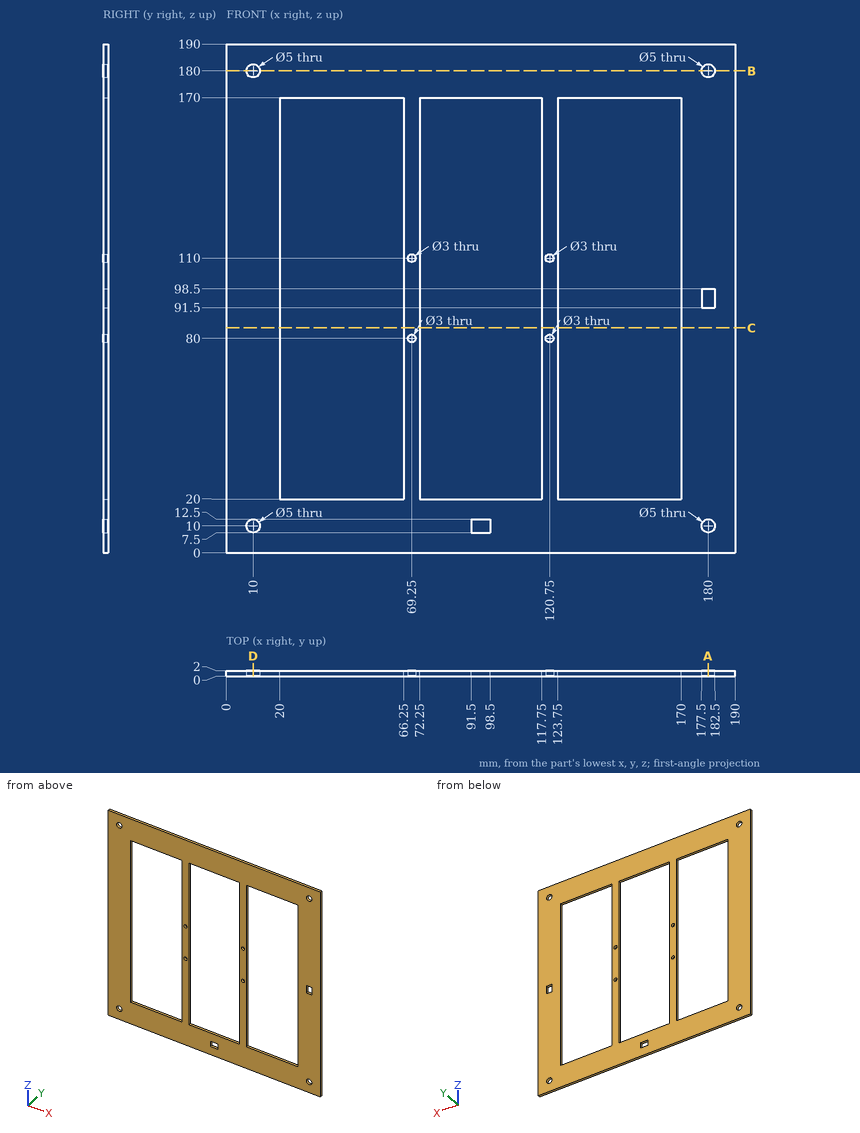
The figure shows three views and two pictorial views of one solid part (mm, origin at its lowest corner). Answer the questions. Give positions to 0.01 mm unless a question says otherwise; leave off trailing zeros. Loops run counter-clockwise (first coordinate to the right, second up) from the corner with the lowest first, then second, coordinate; pieces in that order, holes last. Notation, with made-up numbers: (43.25, -25) -> (75.25, -25) arc R23 cw to (75.25, -2) -> close; hole circle Ø8 at (62, -6.5). An arc over 180 degrees is marked (long way). Use a Markdown table: item, result. Add a question column.
1. Section C-C on z = 84 is taken. Determine the outline of the cut face in (x, y), and give its area (3 significant figures).
2. Find the intervals of material crossed by probe 1 along X at (y, z) = (1.2, 110); probe 2 along X at (y, z) = (1.5, 32); probe 3 along X at (y, z) = (0.2, 10.5), in increasing order.
3. Section B-B on z = 180 is taken. Determine the outline of the cut face in (x, y).
4. A flat-ended cylindrical pin translates along its axis: pin 1 Ø1 at (x, y) = (33, 1.5) entering from -Z. Find the tip coordinate at first contact, or state that the pin passes through.
5. Section A-A on x = 180 is taken. Determine the outline of the cut face in (y, z).
6. Section D-D on x = 10 is taken. Determine the outline of the cut face in (y, z), and give its area (3 significant figures).
Results below:
| question | item | result |
|---|---|---|
| 1 | outline | (0, 0) -> (20, 0) -> (20, 2) -> (0, 2) -> close; (66.25, 0) -> (72.25, 0) -> (72.25, 2) -> (66.25, 2) -> close; (117.75, 0) -> (123.75, 0) -> (123.75, 2) -> (117.75, 2) -> close; (170, 0) -> (190, 0) -> (190, 2) -> (170, 2) -> close |
| 1 | area | 104 mm^2 |
| 2 | probe 1 | x = 0 to 20, 66.25 to 67.75, 70.75 to 72.25, 117.75 to 119.25, 122.25 to 123.75, 170 to 190 |
| 2 | probe 2 | x = 0 to 20, 66.25 to 72.25, 117.75 to 123.75, 170 to 190 |
| 2 | probe 3 | x = 0 to 7.55, 12.45 to 91.5, 98.5 to 177.55, 182.45 to 190 |
| 3 | outline | (0, 0) -> (7.5, 0) -> (7.5, 2) -> (0, 2) -> close; (12.5, 0) -> (177.5, 0) -> (177.5, 2) -> (12.5, 2) -> close; (182.5, 0) -> (190, 0) -> (190, 2) -> (182.5, 2) -> close |
| 4 | pin 1 | stops at z = 0 |
| 5 | outline | (0, 0) -> (2, 0) -> (2, 7.5) -> (0, 7.5) -> close; (0, 12.5) -> (2, 12.5) -> (2, 91.5) -> (0, 91.5) -> close; (0, 98.5) -> (2, 98.5) -> (2, 177.5) -> (0, 177.5) -> close; (0, 182.5) -> (2, 182.5) -> (2, 190) -> (0, 190) -> close |
| 6 | outline | (0, 0) -> (2, 0) -> (2, 7.5) -> (0, 7.5) -> close; (0, 12.5) -> (2, 12.5) -> (2, 177.5) -> (0, 177.5) -> close; (0, 182.5) -> (2, 182.5) -> (2, 190) -> (0, 190) -> close |
| 6 | area | 360 mm^2 |
